Could you check a few things on this model? Use its own coordinates, in mm. A direction names the side the tool comes from. Round coordinates to 2 decimals unless told otherwise and drop trailing zeros. Order: outer loops, then holes, each group sorted by start corner. A loop starts at its lowest first (then second) coordinate and runs counter-clockwise, first axis right, second up. Notation, with made-up numbers: M -11,-15 L 41,-15 A27 ccw 41,23 Z; hole C -22.75,83.25 d8. An arc over 180 degrees is marked long. Write each question's results on one line, items separated by ' | '. Start each with the question number.
1. Please list where these lines run through material, in increasing order: L1, parallel to Z at x = 0, y = 11.6 (3 decimals); L2, parallel to Y at x = 0, z = 4.75; L3, parallel to Z at x = 2, y = -24.
2. Suppose I cut it at C-C on z = 4. Write out the boundary of the cut face in (x, y).
3. For faces 1 (the cylindrical face through (7.724, -12.991, 0.095)), 2 (the cylindrical face through (-7.724, -12.991, -0.141)), 3 (the cylindrical face through (-6.2, 12, 0.9)), 4 (the cylindrical face through (1.25, -27.47, -1.96)), which set-ups out of +Z, -Z, +X, -X, +Y, -Y let a thin tool reach every point of the face, with its end or its side?
4. I'm going to push flat-ended pins straight in: pin 1 (1.4 mm diameter, centred on x = 0, z = 5.45, fed in from -Y); pin 2 (2.5 mm diameter, centred on x = 0, z = -5.45, fed in from +Y); pin 3 (7.5 mm diameter, centred on x = -2, y = -13.5, fed in from -Z). Where does each tip first touch, or does it pass through?
5. We'd pull the mould along X, two halves only. Please class faces 5 (the cylindrical face through (-3, 14, 0)), 6 (the flat face through (0.9, 27, 0)), 7 (the cylindrical face through (6.386, 12.014, 0.575)): released by +X, released by -X, zero draft, split by the parting line, or undercut.
6. Suppose I cut it at B-B on y = -7.5. Write out the boundary of the cut face in (x, z) (3 decimals), and give its area (3 significant figures).
7. Suppose I cut it at D-D on y = 14. Write out the boundary of the cut face in (x, z), and give its area (3 significant figures).
Autodesk Inventor part; units mm, degrees
ref_plane "YZ Plane" through (0, 0, 0) normal (1, 0, 0) x (0, 1, 0)
ref_plane "XZ Plane" through (0, 0, 0) normal (0, 1, 0) x (-1, 0, 0)
ref_plane "XY Plane" through (0, 0, 0) normal (0, 0, 1) x (1, 0, 0)
sketch "Sketch1" plane through (0, 0, 0) normal (0, 1, 0) x (-1, 0, 0)
  circle A0 centre (0, 0) radius 8
  dimension "d0" = 16
extrude "Extrusion1" add sketch "Sketch1" along normal blind 13
sketch "Sketch2" plane through (0, 13, 0) normal (0, 1, 0) x (1, 0, 0)
  circle A0 centre (0, 0) radius 3
  dimension "d3" = 6
extrude "Extrusion2" add sketch "Sketch2" along normal blind 1.85
sketch "Sketch3" plane through (0, 14.85, 0) normal (0, 1, 0) x (1, 0, 0)
  circle A0 centre (0, 0) radius 1.5
  dimension "d6" = 3
extrude "Extrusion3" add sketch "Sketch3" along normal blind 16
sketch "Sketch4" plane through (0, 30.85, 0) normal (0, 1, 0) x (1, 0, 0)
  circle A0 centre (0, 0) radius 1.5
  line L0 (0.9, 0) -> (0.9, 1.2)
  line L1 (0.9, 1.2) -> (0.9, -1.2)
  circle A1 centre (0, 0) radius 3
  arc A2 (0.9, -1.2) -> (0.9, 1.2) centre (0, 0) ccw
extrude "Extrusion4" cut sketch "Sketch4" against normal blind 7 contours A0 L1 L0 picked at (0.9839, 0.7204)
sketch "Sketch5" plane through (0, 13, 0) normal (0, 1, 0) x (1, 0, 0)
  circle A0 centre (5, 0) radius 1.5
  circle A1 centre (-5, 0) radius 1.5
  point P0 (0, 0)
extrude "Extrusion5" cut sketch "Sketch5" against normal blind 2
sketch "Sketch6" plane through (0, 13, 0) normal (0, 1, 0) x (1, 0, 0)
  circle A0 centre (0, 0) radius 8
  circle A1 centre (0, -5.45) radius 0.775
  line L0 (-8, 0) -> (8, 0)
  circle A2 centre (0, 5.45) radius 0.775
extrude "Extrusion6" cut sketch "Sketch6" against normal blind 2 contours A1 | A2
sketch "Sketch7" plane through (0, 13, 0) normal (0, 1, 0) x (1, 0, 0)
  point P0 (0, 0)
sketch "Sketch8" plane through (0, 0, 0) normal (0, -1, 0) x (1, 0, 0)
  circle A0 centre (0, 0) radius 7.725
  dimension "d22" = 15.45
extrude "Extrusion7" add sketch "Sketch8" along normal blind 26.35
sketch "Sketch9" plane through (0, -26.35, 0) normal (0, -1, 0) x (1, 0, 0)
  line L0 (0, -6) -> (-4.8658, -6)
  circle A0 centre (0, 0) radius 7.725
  line L1 (0, -6) -> (4.8658, -6)
  line L2 (0, 6) -> (-4.8653, 6.0004)
  line L3 (0, 6) -> (4.8652, 6.0004)
  arc A1 (-4.8658, -6) -> (4.8658, -6) centre (0, 0) ccw
  arc A2 (4.8652, 6.0004) -> (-4.8653, 6.0004) centre (0, 0) ccw
extrude "Extrusion8" cut sketch "Sketch9" against normal blind 26.35 contours L1 A0 L0 | A0 L3 L2
sketch "Sketch10" plane through (0, -26.35, 0) normal (0, -1, 0) x (1, 0, 0)
  circle A0 centre (0, 0) radius 2.325
  dimension "d29" = 4.65
extrude "Extrusion9" add sketch "Sketch10" along normal blind 2.4
fillet "Fillet1" radius 0.125 1 edges at (-2.325, -28.75, 0)
fillet "Fillet2" radius 0.05 1 edges at (-3, 14.85, 0)
fillet "Fillet3" radius 0.25 3 edges at (4.8658, -13.175, -6) (-4.8653, -13.175, 6.0004) (4.8652, -13.175, 6.0004)
properties part number "Dc Motor 3mm D Shaft"
Filled sheet:
1) L1: z = -8 to -6.225, -4.675 to 4.675, 6.225 to 8 | L2: y = -26.35 to 11 | L3: z = -6 to 6
2) outline: M -6.93,0 L -6.61,0 L -6.61,-26.35 L 6.61,-26.35 L 6.61,0 L 6.93,0 L 6.93,13 L -6.93,13 Z
3) face 1: +X, -Y | face 2: -X, -Y | face 3: +Y | face 4: -Y
4) pin 1: stops at y = -26.35 | pin 2: stops at y = 13 | pin 3: stops at z = -6
5) face 5: split by the parting line | face 6: released by +X | face 7: undercut
6) outline: M -4.936,5.943 A7.725 ccw -4.866,-6 L 4.776,-6 A0.25 ccw 4.936,-5.942 A7.725 ccw 4.936,5.943 A0.25 ccw 4.776,6 L 0,6 L -4.776,6 A0.25 ccw Z | area: 165 mm^2
7) outline: C 0,0 d6 | area: 28.3 mm^2
